Source: CAD feature listing. Evaluate the final solid. Frame: model axes, mm. Face numbers are marked on the shaded views. A direction names the side the tool comes from. Give positions to 0.01 mm unless a question says otherwise; leave off trailing zeros. Loops run counter-clockwise (first coordinate to the right, second up) from the corner with the lowest first, then second, coordinate; pieces in that order, holes last. Notation, with made-up numbers: M 61,77 L 113,77 A19 ccw 113,113 Z; hole C 1.5,-21 d1. An arc over 180 degrees is marked long. Answer in a Markdown table with one row per item.
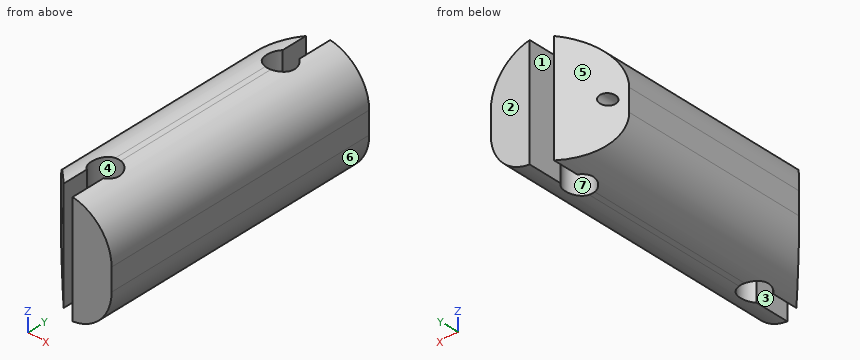
Autodesk Inventor part; units mm, degrees
ref_plane "YZ Plane" through (0, 0, 0) normal (1, 0, 0) x (0, 1, 0)
ref_plane "XZ Plane" through (0, 0, 0) normal (0, 1, 0) x (-1, 0, 0)
ref_plane "XY Plane" through (0, 0, 0) normal (0, 0, 1) x (1, 0, 0)
sketch "Sketch1" plane through (0, 0, 0) normal (0, 0, 1) x (1, 0, 0)
  line L0 (0, 0) -> (2.5, 0)
  line L1 (2.5, 0) -> (2.5, 50)
  line L2 (2.5, 50) -> (-2.5, 50)
  line L3 (-2.5, 50) -> (-2.5, 0)
  circle A0 centre (0, 0) radius 8.5
  line L4 (0, 50) -> (8.5, 50) construction
  circle A1 centre (0, 50) radius 8.5
  line L5 (-8.5, 0) -> (-8.5, 50)
  line L6 (8.5, 50) -> (8.5, 0)
  line L7 (0, 50) -> (8.5, 50)
  line L8 (0, 50) -> (-8.5, 41.5)
  line L9 (0, 50) -> (12.0208, 50) construction
  line L10 (0, 0) -> (8.5, 0)
  line L11 (0, 0) -> (-8.5, 8.5)
  line L12 (0, 0) -> (12.0208, 0) construction
  dimension "d9" = 17
  dimension "d1" = 2.5
  dimension "d2" = 50
  dimension "d3" = 5
  dimension "d5" = 17
  dimension "d10" = 2.5
  dimension "d11" = 0
  dimension "d12" = 135
  dimension "d13" = 135
extrude "Extrusion1" add sketch "Sketch1" along normal blind 20 contours L11 L3 A0 L1 L0 | L1 A0 L10 | L11 A0 L3 | A0 L3 A1 L1 | L1 A1 L6 A0 | A0 L11 L5 L8 A1 L3 | A1 L3 L8 L2 L1 | L1 L7 A1 | A1 L8 L3
sketch "Sketch2" plane through (0, 0, 0) normal (0, 0, -1) x (-1, 0, 0)
  line L0 (0, 0) -> (-8.5, 0)
  line L1 (0, 0) -> (0, 8)
  circle A0 centre (0, 8) radius 2.5
  line L2 (8.5, 8.5) -> (0, 0)
  line L3 (0, 0) -> (-1.5, 0)
  line L4 (-1.5, 0) -> (-1.5, 8)
  line L5 (-1.5, 8) -> (1.5, 8)
  line L6 (1.5, 8) -> (1.5, 0)
  line L7 (1.5, 0) -> (0, 0)
  line L8 (0, 50) -> (8.5, 41.5)
  line L9 (0, 50) -> (0, 42)
  line L10 (0, 42) -> (-1.5, 42)
  line L11 (-1.5, 42) -> (-1.5, 50)
  line L12 (-8.5, 50) -> (0, 50)
  line L13 (0, 42) -> (1.5, 42)
  line L14 (1.5, 42) -> (1.5, 50)
  line L15 (1.5, 50) -> (0, 50)
  circle A1 centre (0, 42) radius 2.5
  point P0 (1.5, 45)
  point P1 (-1.5, 44)
  point P2 (1.5, 44)
  point P3 (-1.5, 6)
  point P4 (1.5, 6)
  dimension "d16" = 8
  dimension "d17" = 5
  dimension "d18" = 1.5
  dimension "d19" = 3
  dimension "d20" = 8
  dimension "d21" = 1.5
  dimension "d22" = 1.5
  dimension "d23" = 5
extrude "Extrusion2" cut sketch "Sketch2" against normal through all
fillet "Fillet1" radius 8 4 edges at (8.5, 25, 0) (8.5, 25, 20) (-8.5, 25, 0) (-8.5, 25, 20)
sketch "Sketch4" plane through (1.5, 0, 0.0627) normal (0, -1, 0) x (1, 0, 0)
  line L0 (-10, 7.9373) -> (-10, 11.9373)
  line L1 (-10, 9.9373) -> (-8, 9.9373)
  circle A0 centre (-8, 9.9373) radius 1
  point P0 (-1.5, -0.0627)
  dimension "d31" = 2
  dimension "d32" = 2
extrude "Extrusion4" cut sketch "Sketch4" against normal through all
properties part number "ring_f1"
Q1. Contact query for flat-ended pins moving along their axis: pin 1 Ø3 at (x, z) = (-6.5, 10) entering from -Y; pin 2 Ø1 at (x, y) = (-5.5, 36.5) entering from +Z; pin 3 Ø3 at (x, y) = (2.5, 25.5) entering from -Z. Output: stop coordinate, or through.
Values follow:
| item | result |
|---|---|
| pin 1 | y = 5 |
| pin 2 | z = 18.61 |
| pin 3 | z = 0.02 |
Q2. Section query B-B (z = 10). Output: boundary loops of the cut face in (x, y), plus the area to 3 significant figures.
Values follow:
| item | result |
|---|---|
| outline | M -8.5,8.5 L -7.5,7.5 L -7.5,42.5 L -8.5,41.5 Z; M -5.5,5.5 L -1.5,1.5 L -1.5,6 A2.5 cw long 1.5,6 L 1.5,0 L 8.5,0 L 8.5,50 L 1.5,50 L 1.5,44 A2.5 cw long -1.5,44 L -1.5,48.5 L -5.5,44.5 Z |
| area | 633 mm^2 |
Q3. Section query D-D (y = 42). Output: boundary loops of the cut face in (x, z), plus the area to 3 significant figures.
Values follow:
| item | result |
|---|---|
| outline | M -8,5.22 A8 ccw -2.5,0.25 L -2.5,19.75 A8 ccw -8,14.78 Z; M 2.5,0.25 A8 ccw 8.5,8 L 8.5,12 A8 ccw 2.5,19.75 Z; hole C -6.5,10 d2 |
| area | 179 mm^2 |
Q4. Reachability of the marked faces 1, 2 and 3 from +Z, -Z, +X, -X, +Y, -Y: full face, straight path, thin tool, end or side. Return the list, or none.
Values follow:
| item | result |
|---|---|
| face 1 | +Z, -Z, +Y |
| face 2 | +Z, -Z, +X, -X, +Y |
| face 3 | +Z, -Z, -Y |
Q5. Section query C-C (x = -6.5). Output: boundary loops of the cut face in (y, z).
Values follow:
| item | result |
|---|---|
| outline | M 6.5,2.71 L 43.5,2.71 L 43.5,9 L 6.5,9 Z; M 6.5,11 L 43.5,11 L 43.5,17.29 L 6.5,17.29 Z |
Q6. Mould query, pull axis X, two halves, no side actions, for the marked faces 4, 5, 6 and 7. Classes: +X half, -X half, draft (parallel to the pull), parting line (faces both ways), or undercut.
Values follow:
| item | result |
|---|---|
| face 4 | undercut |
| face 5 | -X half |
| face 6 | +X half |
| face 7 | undercut |
Q7. Ray query, probe 1 along X at (y, z) = (38.5, 10); probe 2 along Y at (x, z) = (-0.5, 6.5); probe 3 along X at (y, z) = (8, 10.75). Return the intervals inside material, ascending. Write a range as from..to.
Values follow:
| item | result |
|---|---|
| probe 1 | -8.5..-7.5, -5.5..8.5 |
| probe 2 | 10.45..39.55 |
| probe 3 | -8..-7.16, -5.84..-2.5, 2.5..8.5 |
Q8. Section query A-A (y = 20). Output: boundary loops of the cut face in (x, z), plus the area to 3 significant figures.
Values follow:
| item | result |
|---|---|
| outline | M -8.5,8 A8 ccw -0.5,0 L 0.5,0 A8 ccw 8.5,8 L 8.5,12 A8 ccw 0.5,20 L -0.5,20 A8 ccw -8.5,12 Z; hole C -6.5,10 d2 |
| area | 282 mm^2 |
